```python
from build123d import *

# Parameters (mm, degrees)
SKETCH1_W                                          = 114.3
SKETCH1_H                                          = 88.9
SKETCH1_W_2                                        = 101.6
SKETCH1_H_2                                        = 76.2
BOSS_EXTRUDE1_DEPTH                                = 12.7
SKETCH2_W                                          = 114.3
SKETCH2_H                                          = 88.9
BOSS_EXTRUDE2_DEPTH                                = 6.35
FILLET1_R                                          = 12.7
CUT_EXTRUDE1_REACH                                 = 108.445
FILLET2_R                                          = 3.175
CSK_FOR_10_FLAT_HEAD_MACHINE_SCREW_100_D           = 5.1054
CSK_FOR_10_FLAT_HEAD_MACHINE_SCREW_100_CSINK_D     = 9.779
CSK_FOR_10_FLAT_HEAD_MACHINE_SCREW_100_CSINK_ANGLE = 100
CHAMFER1_SIZE                                      = 1.407761108
CHAMFER1_SIZE_2                                    = 6.35


with BuildPart() as part:
    # Sketch1 → Boss-Extrude1 (new body)
    with BuildSketch(Plane(origin=(0, 0, 0), x_dir=(1, 0, 0), z_dir=(0, 1, 0))):
        Rectangle(SKETCH1_W, SKETCH1_H)
        Rectangle(SKETCH1_W_2, SKETCH1_H_2, mode=Mode.SUBTRACT)
    extrude(amount=BOSS_EXTRUDE1_DEPTH)

    # Sketch2 → Boss-Extrude2 (add)
    with BuildSketch(Plane.XZ):
        Rectangle(SKETCH2_W, SKETCH2_H)
    extrude(amount=BOSS_EXTRUDE2_DEPTH)

    # Fillet1
    fillet1_edges = [part.edges().sort_by_distance(p)[0] for p in [
        (50.8, 6.35, 38.1),
        (50.8, 6.35, -38.1),
        (-50.8, 6.35, -38.1),
        (-50.8, 6.35, 38.1),
        (-57.15, 3.175, 44.45),
        (-57.15, 3.175, -44.45),
        (57.15, 3.175, -44.45),
        (57.15, 3.175, 44.45),
    ]]
    fillet(fillet1_edges, radius=FILLET1_R)

    # Sketch3 → Cut-Extrude1 (cut, up to next)
    with BuildSketch(Plane(origin=(0, 0, -44.45), x_dir=(-1, 0, 0), z_dir=(0, 0, -1)), mode=Mode.PRIVATE) as cut_extrude1_sk1:
        with BuildLine():
            Line((2.54, 22.86), (2.54, 2.54))
            ThreePointArc((2.54, 2.54), (0, 0), (-2.54, 2.54))
            Line((-2.54, 2.54), (-2.54, 22.86))
            ThreePointArc((-2.54, 22.86), (0, 25.4), (2.54, 22.86))
        make_face()
    cut_extrude1_tool1 = extrude(cut_extrude1_sk1.sketch, amount=-CUT_EXTRUDE1_REACH, mode=Mode.PRIVATE) & part.part
    add(cut_extrude1_tool1.solids().sort_by_distance((0, 12.7, -44.45))[0], mode=Mode.SUBTRACT)

    # Fillet2
    fillet2_edges = [part.edges().sort_by_distance(p)[0] for p in [
        (2.54, 12.7, -41.275),
        (-2.54, 12.7, -41.275),
    ]]
    fillet(fillet2_edges, radius=FILLET2_R)

    # CSK for #10 Flat Head Machine Screw (100)1 (through all)
    with Locations(Plane(origin=(0, 0, 0), x_dir=(1, 0, 0), z_dir=(0, 1, 0))):
        with Locations((0, 0)):
            CounterSinkHole(CSK_FOR_10_FLAT_HEAD_MACHINE_SCREW_100_D / 2, CSK_FOR_10_FLAT_HEAD_MACHINE_SCREW_100_CSINK_D / 2, counter_sink_angle=CSK_FOR_10_FLAT_HEAD_MACHINE_SCREW_100_CSINK_ANGLE)

    # Chamfer1
    # the kernel refuses this chamfer: 6.35, 1.407761108 mm, written as the material it takes off along each edge
    with BuildSketch(Plane(origin=(-44.45, 12.7, -44.45), x_dir=(0, 0.16714603522124954, 0.9859321492424399), z_dir=(1, 0, 0)), Plane(origin=(-10.78052054, 12.7, -44.45), x_dir=(0, 0.16714603522124954, 0.9859321492424399), z_dir=(1, 0, 0))) as chamfer1_piece_1:
        Polygon((CHAMFER1_SIZE * 0.98593214909, CHAMFER1_SIZE * 0.167146035195), (-CHAMFER1_SIZE_2 * 0.167146035221, CHAMFER1_SIZE_2 * 0.985932149242), (0, 0), align=None)
    extrude(amount=55.23052054, mode=Mode.SUBTRACT)
    with BuildSketch(Plane(origin=(57.15, 12.7, -31.75), x_dir=(-0.9859321492424399, 0.16714603522124954, 0), z_dir=(0, 0, 1)), Plane(origin=(-57.15, 12.7, 31.75), x_dir=(0.9859321492424399, 0.16714603522124954, 0), z_dir=(0, 0, -1))) as chamfer1_piece_2:
        Polygon((CHAMFER1_SIZE * 0.98593214909, CHAMFER1_SIZE * 0.167146035195), (-CHAMFER1_SIZE_2 * 0.167146035221, CHAMFER1_SIZE_2 * 0.985932149242), (0, 0), align=None)
    extrude(amount=63.5, mode=Mode.SUBTRACT)
    with BuildSketch(Plane(origin=(44.45, 12.7, 44.45), x_dir=(0, 0.16714603522124954, -0.9859321492424399), z_dir=(-1, 0, 0))) as chamfer1_piece_3:
        Polygon((CHAMFER1_SIZE * 0.98593214909, CHAMFER1_SIZE * 0.167146035195), (-CHAMFER1_SIZE_2 * 0.167146035221, CHAMFER1_SIZE_2 * 0.985932149242), (0, 0), align=None)
    extrude(amount=88.9, mode=Mode.SUBTRACT)
    with BuildSketch(Plane(origin=(44.45, 12.7, -31.75), x_dir=(1, 0, 0), z_dir=(0, 0, 1))) as chamfer1_piece_4:
        Polygon((12.7 - CHAMFER1_SIZE, 0), (12.7, -CHAMFER1_SIZE_2), (12.7, 0), align=None)
    revolve(axis=Axis((44.45, 12.7, -31.75), (0, 1, 0)), revolution_arc=90, mode=Mode.SUBTRACT)
    with BuildSketch(Plane(origin=(-44.45, 12.7, -31.75), x_dir=(-1, 0, 0), z_dir=(0, 0, 1))) as chamfer1_piece_5:
        Polygon((12.7 - CHAMFER1_SIZE, 0), (12.7, CHAMFER1_SIZE_2), (12.7, 0), align=None)
    revolve(axis=Axis((-44.45, 12.7, -31.75), (0, -1, 0)), revolution_arc=90, mode=Mode.SUBTRACT)
    with BuildSketch(Plane(origin=(-44.45, 12.7, 31.75), x_dir=(-1, 0, 0), z_dir=(0, 0, -1))) as chamfer1_piece_6:
        Polygon((12.7 - CHAMFER1_SIZE, 0), (12.7, -CHAMFER1_SIZE_2), (12.7, 0), align=None)
    revolve(axis=Axis((-44.45, 12.7, 31.75), (0, 1, 0)), revolution_arc=90, mode=Mode.SUBTRACT)
    with BuildSketch(Plane(origin=(44.45, 12.7, 31.75), x_dir=(0, 0, 1), z_dir=(-1, 0, 0))) as chamfer1_piece_7:
        Polygon((12.7 - CHAMFER1_SIZE, 0), (12.7, -CHAMFER1_SIZE_2), (12.7, 0), align=None)
    revolve(axis=Axis((44.45, 12.7, 31.75), (0, 1, 0)), revolution_arc=90, mode=Mode.SUBTRACT)


solid = part.part
```
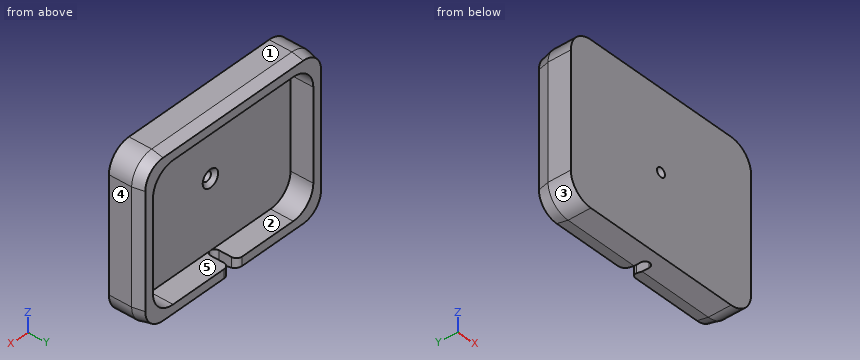
Geometry check sheet. Reference: the model listing, model coordinates, mm. Face numbers are marked on the shaded views. A direction names the side the tool comes from. Give positions to 0.01 mm unless a question says otherwise; leave off trailing zeros. Order: outer loops, then holes, each group sorted by start corner. A loop starts at its lowest first (then second) coordinate and runs counter-clockwise, first axis right, second up. Notation, with made-up numbers: (-39, -15) - (-25, -15) arc R31 ccw to (-25, 20) - close; hole circle Ø10 at (59, 85). An arc over 180 degrees is marked (long way). Write item = value, one per line. Start each with the question number.
1) Section check B-B (x = -23.5). Enter the section's corners in (y, z), then the cut area to 3 significant figures.
2) Draft check along X on the marked faces 3, 4 and 5. Enter one of: released by +X, released by -X, zero draft, split by the parting line, or undercut.
3) Access from +Z, -Z, +X, -X, +Y, -Y to the whole of each face (thin tool, end or side, straight path). Record for the marked faces 1 and 2.
4) Section check C-C (x = -40). Enter the section's corners in (y, z), then the cut area to 3 significant figures.
5) Gauge pin test, flat ends, axial feed: pin 1 Ø5 at (y, z) = (6.5, -41.5) entering from -X; pin 2 Ø6 at (x, z) = (0, 0) entering from +Y; pin 3 Ø1.5 at (x, z) = (-41, 28) entering from +Y. Record the tip position at first contact, or that the pin passes through.
6) Section check A-A (z = 0). Enter the section's corners in (x, y), then the cut area to 3 significant figures.
7) Scan lines: L1, parallel to Z at x = 35.5, y = 2; L2, parallel to X at y = 3.75, z = 10; L3, parallel to Z at x = 0, y = -4.65. Record each from-to range of solid material in increasing order.
Geometry check:
q1.outline = (-6.35, -44.45) - (6.35, -44.45) - (12.7, -43.04) - (12.7, -38.1) - (0, -38.1) - (0, 38.1) - (12.7, 38.1) - (12.7, 43.04) - (6.35, 44.45) - (-6.35, 44.45) - close
q1.area = 717 mm2
q2.face_3 = released by -X
q2.face_4 = released by +X
q2.face_5 = undercut
q3.face_1 = +Z, +X, -X, +Y, -Y
q3.face_2 = +Y
q4.outline = (-6.35, -44.45) - (6.35, -44.45) - (12.7, -43.04) - (12.7, -37.96) - (0, -37.96) - (0, 37.96) - (12.7, 37.96) - (12.7, 43.04) - (6.35, 44.45) - (-6.35, 44.45) - close
q4.area = 720 mm2
q5.pin_1 = -54.87
q5.pin_2 = -1.59
q5.pin_3 = 0
q6.outline = (-57.15, -6.35) - (-2.55, -6.35) - (-2.55, -1.96) - (-4.89, 0) - (-50.8, 0) - (-50.8, 12.7) - (-55.74, 12.7) - (-57.15, 6.35) - close; (2.55, -6.35) - (57.15, -6.35) - (57.15, 6.35) - (55.74, 12.7) - (50.8, 12.7) - (50.8, 0) - (4.89, 0) - (2.55, -1.96) - close
q6.area = 841 mm2
q7.L1 = -44.45 to -38.1, 38.1 to 44.45
q7.L2 = -57.15 to -50.8, 50.8 to 57.15
q7.L3 = -44.45 to -2.55, 2.55 to 44.45
